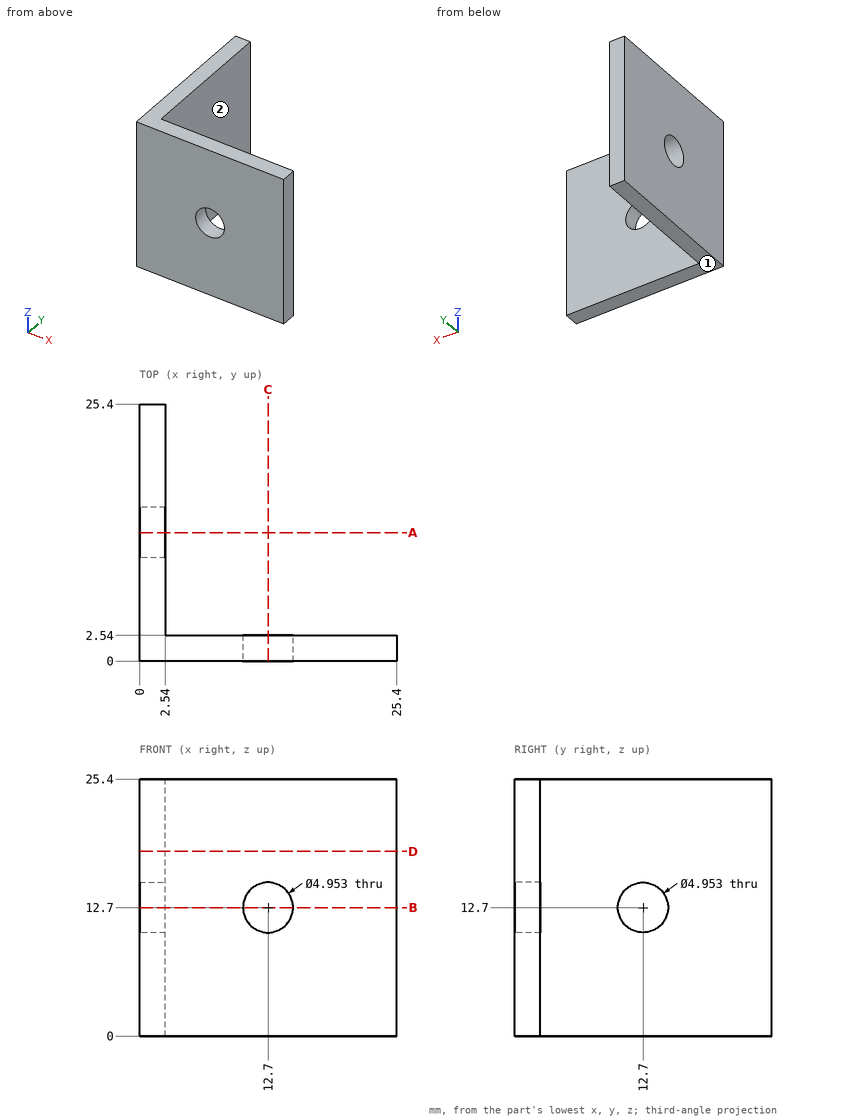
Here's the drawing with two shaded views (mm, measured from the low corner). I have some questions. A direction names the side the tool comes from. Coordinates: 2 decimals unless noted, no trailing zeros. Loops run counter-clockwise (first coordinate to the right, second up) from the corner with the lowest first, then second, coordinate; pieces in that order, holes last. Notation, with made-up numbers: (86, 63.5) -> (138, 63.5) arc R17 cw to (138, 95.5) -> close; hole circle Ø2 at (73.5, 52). An arc over 180 degrees is marked (long way). Answer as a JSON object with one key per item and string values.
1) If I drill on line 1 (Y direction, x = 10.5, z = 11.5); line 2 (Y direction, x = 1.75, z = 12.7), over which ranges is the centre line in solid material (lowest first)?
Results:
{"line 1": "y = 0 to 2.54", "line 2": "y = 0 to 10.22, 15.18 to 25.4"}
2) Imagine slicing it at A-A (y = 12.7). Please give me the cut outline in (x, z).
Results:
{"outline": "(0, 0) -> (2.54, 0) -> (2.54, 10.22) -> (0, 10.22) -> close; (0, 15.18) -> (2.54, 15.18) -> (2.54, 25.4) -> (0, 25.4) -> close"}
3) Imagine slicing it at D-D (z = 18.25). Please give me the cut outline in (x, y), then the cut area to 3 significant figures.
Results:
{"outline": "(0, 0) -> (25.4, 0) -> (25.4, 2.54) -> (2.54, 2.54) -> (2.54, 25.4) -> (0, 25.4) -> close", "area": "123 mm^2"}
4) For P1, Ø8, axis at y = 8, z = 15.5, coming from the +X side; P2, Ø6.5, axis at x = 12.7, z = 12.7, coming from the +Y side, each with a flat end and sliding along its axis, tell me the tip position at first contact or that it passes through.
Results:
{"P1": "stops at x = 2.54", "P2": "stops at y = 2.54"}
5) For the marked faces 1 and 2, which set-ups out of +Z, -Z, +X, -X, +Y, -Y let a thin tool reach every point of the face, with its end or its side?
Results:
{"face 1": "-Z, +X, -X, +Y, -Y", "face 2": "+Z, -Z, +X, +Y"}
6) Imagine slicing it at B-B (z = 12.7). Please give me the cut outline in (x, y), then the cut area to 3 significant figures.
Results:
{"outline": "(0, 0) -> (10.22, 0) -> (10.22, 2.54) -> (2.54, 2.54) -> (2.54, 10.22) -> (0, 10.22) -> close; (0, 15.18) -> (2.54, 15.18) -> (2.54, 25.4) -> (0, 25.4) -> close; (15.18, 0) -> (25.4, 0) -> (25.4, 2.54) -> (15.18, 2.54) -> close", "area": "97.4 mm^2"}
